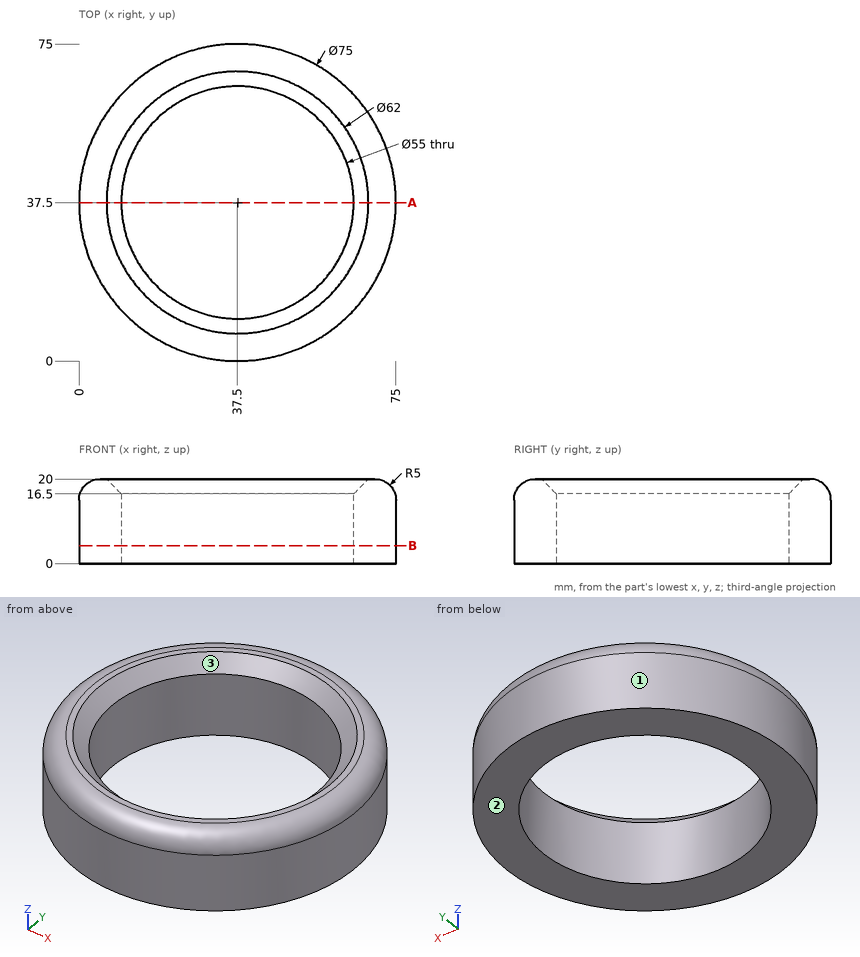
Check sheet for the drawn part. Datum: minimum x, y, z corner. Units: mm. Give positions to 0.01 mm unless a question says otherwise; leave off trailing zeros. Write each loop counter-clockwise with the first axis right and the second up, starting at its lowest first coordinate (ties: lowest second). Pieces come first, ordered by that corner, then holes. Notation, with made-up numbers: (52.5, 8) -> (89.5, 8) arc R25 cw to (89.5, 26) -> close; hole circle Ø4 at (4, -9). An arc over 180 degrees is marked (long way). Use one line per item in the form item = value. Start each with the question number.
1. Section check B-B (z = 4.25). Record the cut outline in (x, y).
2. Mould release check, pull along X, two halves, no side actions. Record for the marked faces 1, 2 and 3: pulls with the +X half, pulls with the -X half, needs draft (parallel to the pull), parting line crosses it, or undercut.
3. Section check A-A (y = 37.5). Record the cut outline in (x, z).
4. Go/stop test with flat-tipped pins: P1, Ø1, axis at x = 30.5, z = 17, coming from the +Y side; P2, Ø3, axis at x = 40.5, z = 13, coming from the +Y side; P3, Ø8, axis at x = 21, y = 21, coming from the +Z side; P4, Ø12, axis at y = 61.5, z = 16, coming from the -X side. Record where each tip stops, or that it passes through.
5. Thickness scan on line 1 along Y through (x, z) = (37.5, 6.5); line 2 along X through (y, z) = (61.5, 2.5); line 3 along X through (y, z) = (53, 3.25). Record the ranges inside material, lowest first. Write a range as from..to.
Conclusion:
q1.outline = circle Ø75 at (37.5, 37.5); hole circle Ø55 at (37.5, 37.5)
q2.face_1 = parting line crosses it
q2.face_2 = needs draft
q2.face_3 = undercut
q3.outline = (0, 0) -> (10, 0) -> (10, 16.5) -> (6.5, 20) -> (5, 20) arc R5 ccw to (0, 15) -> close; (65, 0) -> (75, 0) -> (75, 15) arc R5 ccw to (70, 20) -> (68.5, 20) -> (65, 16.5) -> close
q4.P1 = 74.13
q4.P2 = 74.97
q4.P3 = through
q4.P4 = 4.64
q5.line_1 = 0..10, 65..75
q5.line_2 = 8.69..24.07, 50.93..66.31
q5.line_3 = 3.35..14.78, 60.22..71.65
